from build123d import *

# Parameters (mm, degrees)
SKETCH1_R           = 87.5
BOSS_EXTRUDE1_DEPTH = 120
CUT_EXTRUDE1_DEPTH  = 10
CIRPATTERN1_COUNT   = 8
CUT_EXTRUDE2_DEPTH  = 10
CIRPATTERN2_COUNT   = 8
SKETCH5_R           = 15
CUT_EXTRUDE3_DEPTH  = 121


with BuildPart() as part:
    # Sketch1 → Boss-Extrude1 (new body)
    with BuildSketch(Plane.XY):
        Circle(SKETCH1_R)
    extrude(amount=BOSS_EXTRUDE1_DEPTH)

    # Sketch2 → Cut-Extrude1 (cut)
    with BuildSketch(Plane.XY.offset(120)):
        Polygon((-104.60287609, 492.11784039), (-18.192272947, 85.587915064), (0, 0), (18.192272947, 85.587915064), (104.60287609, 492.11784039), (104.60287609, 1323.341931767), (-104.60287609, 1323.341931767), align=None)
    cut_extrude1 = extrude(amount=-CUT_EXTRUDE1_DEPTH, mode=Mode.SUBTRACT)

    # CirPattern1: Cut-Extrude1 ×8 about axis
    cirpattern1_axis = Axis((0, -4.136271665, 0), (0, 0, 1))
    for i in range(1, CIRPATTERN1_COUNT):
        add(cut_extrude1.rotate(cirpattern1_axis, i * 360 / CIRPATTERN1_COUNT), mode=Mode.SUBTRACT)

    # Sketch4 → Cut-Extrude2 (cut)
    with BuildSketch(Plane(origin=(0, 0, 0), x_dir=(-1, 0, 0), z_dir=(0, 0, -1))):
        Polygon((-109.002412997, 491.678111226), (-18.93846622, 85.425900623), (0, 0), (18.93846622, 85.425900623), (109.002412997, 491.678111226), (109.002412997, 1323.909745158), (-109.002412997, 1323.909745158), align=None)
    cut_extrude2 = extrude(amount=-CUT_EXTRUDE2_DEPTH, mode=Mode.SUBTRACT)

    # CirPattern2: Cut-Extrude2 ×8 about axis
    cirpattern2_axis = Axis((0, -4.318782825, 0), (0, 0, 1))
    for i in range(1, CIRPATTERN2_COUNT):
        add(cut_extrude2.rotate(cirpattern2_axis, i * 360 / CIRPATTERN2_COUNT), mode=Mode.SUBTRACT)

    # Sketch5 → Cut-Extrude3 (cut, through all)
    with BuildSketch(Plane.XY.offset(120)):
        Circle(SKETCH5_R)
    extrude(amount=-CUT_EXTRUDE3_DEPTH, mode=Mode.SUBTRACT)


solid = part.part
Geometry: final body of the model. Coordinates: model frame, mm. A direction names the side the tool comes from. Coordinates: 2 decimals unless noted, no trailing zeros. Order: outer loops, then holes, each group sorted by start corner. A loop starts at its lowest first (then second) coordinate and runs counter-clockwise, first axis right, second up.
1) Section D-D (x = -62). Return loops of the section in (y, z).
Result sheet:
outline: (-61.74, 10) - (-44.93, 10) - (-44.93, 0) - (-17.11, 0) - (-17.11, 10) - (8.47, 10) - (8.47, 0) - (36.29, 0) - (36.29, 10) - (61.74, 10) - (61.74, 110) - (37.15, 110) - (37.15, 120) - (8.16, 120) - (8.16, 110) - (-16.44, 110) - (-16.44, 120) - (-45.42, 120) - (-45.42, 110) - (-61.74, 110) - close
2) Draft query along Y for faces 1 (the flat face through (-10.76, 50.63, 115.07)), 2 (the flat face through (26.621, -44.365, 4.93)), 3 (the flat face through (21, 57, 120)). Return one class per face: released by +Y, released by -Y, zero draft, split by the parting line, or undercut.
Result sheet:
face 1: released by +Y
face 2: undercut
face 3: zero draft
3) Set-up query: faces 4 (the flat face through (-51.13, 6.06, 4.93)), 5 (the flat face through (50.13, 5.837, 4.93)), 6 (the flat face through (-39.88, -31.06, 115.07)). Return all of +Z, -Z, +X, -X, +Y, -Y with unobstructed straight access to the full face (end or side cutting, diameter ignored); none if empty.
Result sheet:
face 4: -Z, -X
face 5: -Z, +X
face 6: +Z
4) Section B-B (z = 76). Return loops of the section in (x, y).
Result sheet:
outline: circle Ø175 at (0, 0); hole circle Ø30 at (0, 0)
5) First-contact query: P1, Ø4, axis at x = -3, z = 103, coming from the -Y side; P2, Ø12, axis at y = -69.5, z = 93, coming from the +X side; P3, Ø10, axis at x = -46.5, z = 53, coming from the +Y side. Flat tips, straight axial feed; report the tip coordinate or a pass-through.
Result sheet:
P1: stops at y = -87.49
P2: stops at x = 60.2
P3: stops at y = 77.03
6) Ray query, probe 1 along Y at (x, z) = (0, 83); probe 2 along Z at (x, y) = (-42, -57). Return the intervals inside material, ascending.
Result sheet:
probe 1: y = -87.5 to -15, 15 to 87.5
probe 2: z = 10 to 110
7) Section A-A (x = -22.5). Return loops of the section in (y, z), then the cut area to 3 significant figures.
Result sheet:
outline: (-84.56, 0) - (-37.9, 0) - (-37.9, 10) - (-19.76, 10) - (-19.76, 0) - (-8.35, 0) - (-8.35, 10) - (-0.29, 10) - (-0.29, 0) - (11.12, 0) - (11.12, 10) - (29.26, 10) - (29.26, 0) - (84.56, 0) - (84.56, 120) - (28.93, 120) - (28.93, 110) - (11.5, 110) - (11.5, 120) - (-0.23, 120) - (-0.23, 110) - (-8.04, 110) - (-8.04, 120) - (-19.77, 120) - (-19.77, 110) - (-37.2, 110) - (-37.2, 120) - (-84.56, 120) - close
area: 19,400 mm2
8) Section C-C (y = -43). Return loops of the section in (x, z).
Result sheet:
outline: (-76.21, 0) - (-58.98, 0) - (-58.98, 10) - (-25.75, 10) - (-25.75, 0) - (-7.62, 0) - (-7.62, 10) - (7.62, 10) - (7.62, 0) - (25.75, 0) - (25.75, 10) - (58.98, 10) - (58.98, 0) - (76.21, 0) - (76.21, 120) - (58.27, 120) - (58.27, 110) - (26.26, 110) - (26.26, 120) - (7.38, 120) - (7.38, 110) - (-7.38, 110) - (-7.38, 120) - (-26.26, 120) - (-26.26, 110) - (-58.27, 110) - (-58.27, 120) - (-76.21, 120) - close
